from build123d import *

# Parameters (mm, degrees)
F0_W     = 50
F0_H     = 50
F1_DEPTH = 4
F2_W     = 43.4
F2_H     = 43.4
F3_DEPTH = 3
F4_R     = 3
F5_DEPTH = 25
F6_R     = 5
F6_R_2   = 3
F7_DEPTH = 3
F8_R     = 3


# Not quite as in the source:
# - a feature names something its author has since deleted; it is built from what else it names


with BuildPart() as f1:
    # F0 (on Front) → F1 (new body)
    with BuildSketch(Plane.XZ):
        Rectangle(F0_W, F0_H)
    extrude(amount=-F1_DEPTH)

    # F2 (on face) → F3 (join)
    with BuildSketch(Plane(origin=(0, 4, 0), x_dir=(-1, 0, 0), z_dir=(0, 1, 0))):
        Rectangle(F2_W, F2_H)
    extrude(amount=F3_DEPTH)

    # F4 (on face) → F5 (cut)
    with BuildSketch(Plane(origin=(0, 7, 0), x_dir=(-1, 0, 0), z_dir=(0, 1, 0))):
        with Locations((-16.5, 16.5)):
            Circle(F4_R)
        with Locations((16.5, 16.5)):
            Circle(F4_R)
        with Locations((16.5, -16.5)):
            Circle(F4_R)
        with Locations((-16.5, -16.5)):
            Circle(F4_R)
    extrude(amount=-F5_DEPTH, mode=Mode.SUBTRACT)

    # F6 (on face) → F7 (cut)
    with BuildSketch(Plane.XZ):
        with Locations((-16.5, 16.5)):
            Circle(F6_R)
        with Locations((-16.5, 16.5)):
            Circle(F6_R_2, mode=Mode.SUBTRACT)
        with Locations((16.5, 16.5)):
            Circle(F6_R)
        with Locations((16.5, 16.5)):
            Circle(F6_R_2, mode=Mode.SUBTRACT)
        with Locations((16.5, -16.5)):
            Circle(F6_R)
        with Locations((16.5, -16.5)):
            Circle(F6_R_2, mode=Mode.SUBTRACT)
        with Locations((-16.5, -16.5)):
            Circle(F6_R)
        with Locations((-16.5, -16.5)):
            Circle(F6_R_2, mode=Mode.SUBTRACT)
    extrude(amount=-F7_DEPTH, mode=Mode.SUBTRACT)

    # F8
    f8_edges = [f1.edges().sort_by_distance(p)[0] for p in [
        (21.7, 5.5, 21.7),
        (-21.7, 5.5, 21.7),
        (-21.7, 5.5, -21.7),
        (21.7, 5.5, -21.7),
    ]]
    fillet(f8_edges, radius=F8_R)


solid = f1.part
Source: CAD feature listing. Evaluate the final solid. Frame: model axes, mm. A direction names the side the tool comes from. Round coordinates to 2 decimals unless told otherwise and drop trailing zeros. Loops run counter-clockwise (first coordinate to the right, second up) from the corner with the lowest first, then second, coordinate; pieces in that order, holes last.
Q1. Access query for faces 1 (the face through (20.8, 5.52, -20.84)), 2 (the face through (-23, 4, 0)), 3 (the face through (-21.7, 5, 0)), 4 (the face through (18.807, 1.479, 12.064)). Directions: +Z, -Z, +X, -X, +Y, -Y. A direction counts if a zero-diameter tool reaches every point of the face in a straight line with its end or side. Return the directions, or none.
Q2. First-contact query: P1, Ø7, axis at x = -16.5, z = 16.5, coming from the -Y side; P2, Ø5.5, axis at x = 16.5, z = 16.5, coming from the -Y side; P3, Ø0.9, axis at y = 6, z = -8, coming from the +X side. Flat tips, straight axial feed; report the tip coordinate or a pass-through.
Q3. Section A-A, the plane x = -16.5. Return loops of the section in (y, z), plus the area to 3 significant figures.
Q4. Section D-D, the plane z = -6. Return loops of the section in (x, y).
Q5. Section C-C, the plane z = 16.5. Return loops of the section in (x, y).
Q6. Mould query, pull axis Z, two halves, no side actions, for faces 5 (the face through (18.9, 5, 14.7)), 6 (the face through (20.8, 5.52, 20.84)), 7 (the face through (0, 0, 0)), 8 (the face through (-17.58, 1.48, 11.62)). Classes: pulls with the +Z half, pulls with the -Z half, needs draft (parallel to the pull), parting line crosses it, or undercut.
Q7. Ray query, line 1 (Z direction, x = 16.5, y = 0.95); line 2 (Z direction, x = 16.5, y = 6.25); line 3 (X direction, y = 4.5, z = -19). Return the intervals inside material, ascending.
Q8. Section B-B, the plane y = 5.5. Return loops of the section in (x, z).
Solutions:
1. face 1: -Z, +X, +Y
1. face 2: +Y
1. face 3: +Z, -Z, -X, +Y
1. face 4: -Y
2. P1: stops at y = 3
2. P2: passes through
2. P3: stops at x = 21.7
3. outline: (0, -25) - (4, -25) - (4, -21.7) - (7, -21.7) - (7, -19.5) - (3, -19.5) - (3, -21.5) - (0, -21.5) - close; (0, -11.5) - (3, -11.5) - (3, -13.5) - (7, -13.5) - (7, 13.5) - (3, 13.5) - (3, 11.5) - (0, 11.5) - close; (0, 21.5) - (3, 21.5) - (3, 19.5) - (7, 19.5) - (7, 21.7) - (4, 21.7) - (4, 25) - (0, 25) - close
3. area: 222 mm2
4. outline: (-25, 0) - (25, 0) - (25, 4) - (21.7, 4) - (21.7, 7) - (-21.7, 7) - (-21.7, 4) - (-25, 4) - close
5. outline: (-25, 0) - (-21.5, 0) - (-21.5, 3) - (-19.5, 3) - (-19.5, 7) - (-21.7, 7) - (-21.7, 4) - (-25, 4) - close; (-13.5, 3) - (-11.5, 3) - (-11.5, 0) - (11.5, 0) - (11.5, 3) - (13.5, 3) - (13.5, 7) - (-13.5, 7) - close; (19.5, 3) - (21.5, 3) - (21.5, 0) - (25, 0) - (25, 4) - (21.7, 4) - (21.7, 7) - (19.5, 7) - close
6. face 5: undercut
6. face 6: pulls with the +Z half
6. face 7: needs draft
6. face 8: undercut
7. line 1: z = -25 to -21.5, -11.5 to 11.5, 21.5 to 25
7. line 2: z = -21.7 to -19.5, -13.5 to 13.5, 19.5 to 21.7
7. line 3: x = -21.68 to -18.16, -14.84 to 14.84, 18.16 to 21.68
8. outline: (-21.7, -18.7) arc R3 ccw to (-18.7, -21.7) - (18.7, -21.7) arc R3 ccw to (21.7, -18.7) - (21.7, 18.7) arc R3 ccw to (18.7, 21.7) - (-18.7, 21.7) arc R3 ccw to (-21.7, 18.7) - close; hole circle Ø6 at (-16.5, -16.5); hole circle Ø6 at (-16.5, 16.5); hole circle Ø6 at (16.5, -16.5); hole circle Ø6 at (16.5, 16.5)
